Could you check a few things on this drawing? It's one solid part, dimensions in mm from its lowest x, y, z. Round coordinates to 2 decimals unless told otherwise and drop trailing zeros. Order: outer loops, then holes, each group sorted by start corner. A loop starts at its lowest first (then second) coordinate and runs counter-clockwise, first axis right, second up. Notation, with made-up numbers: (61.25, 0.25) - (89.25, 0.25) arc R26 ccw to (89.25, 18.25) - close; hole circle Ø3 at (0.5, 27). An arc over 180 degrees is marked (long way). Use one line per item in the form item = value.
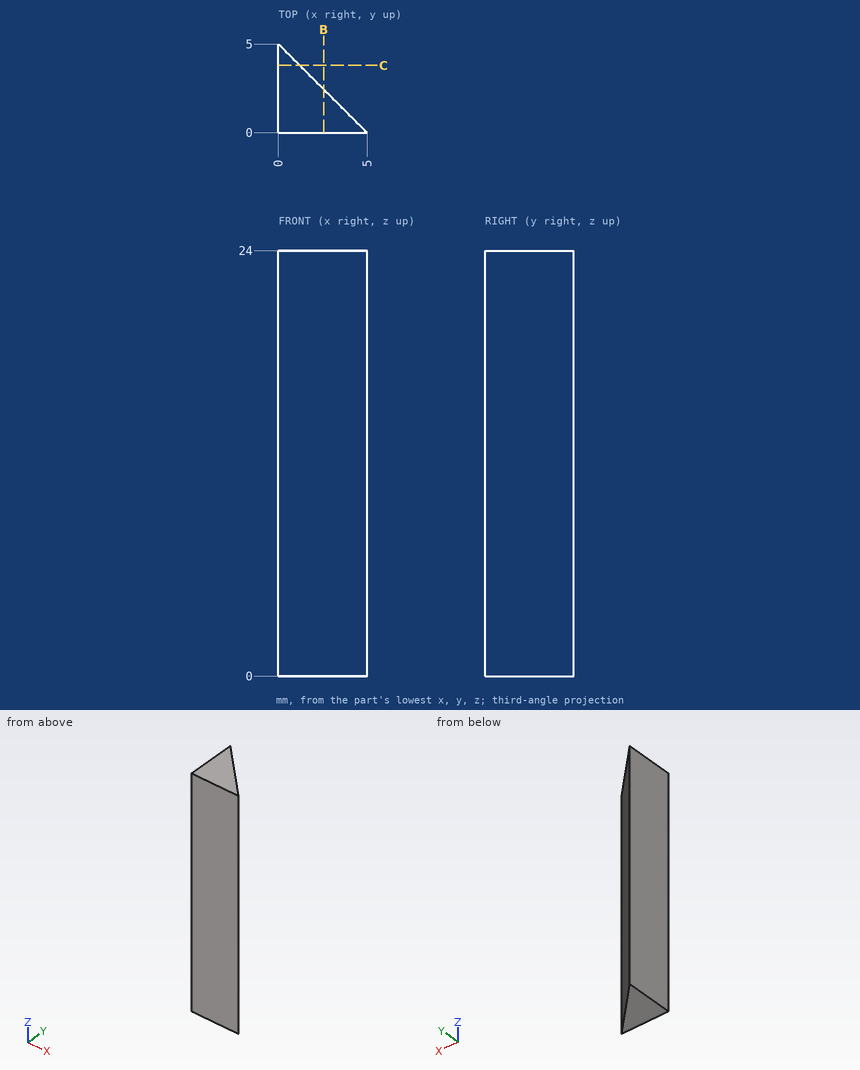
Item 1: Imagine slicing it at C-C on y = 3.8. Please give me the cut outline in (x, z).
Found:
outline = (0, 0) - (1.2, 0) - (1.2, 24) - (0, 24) - close
Item 2: Will these pins go through, and if not, where does the flat tip stop? P1, Ø3, axis at y = 1.5, z = 13.5, coming from the -X side; P2, Ø1, axis at x = 3, z = 13.5, coming from the +Y side.
Found:
P1 = 0
P2 = 2.5
Item 3: I need wall thicknesses on L1, parallel to X at y = 4.5, z = 2; L2, parallel to X at y = 3.8, z = 19.5; L3, parallel to Y at x = 1.25, z = 14.75. Which ranges of each line are inside material? Lowest first, please.
Found:
L1 = 0 to 0.5
L2 = 0 to 1.2
L3 = 0 to 3.75
Item 4: Imagine slicing it at B-B on x = 2.55. Please give me the cut outline in (y, z), plus the area to 3 significant figures.
Found:
outline = (0, 0) - (2.45, 0) - (2.45, 24) - (0, 24) - close
area = 58.8 mm2
